For this review, use the dimensioned drawing (mm, ordinates from the lowest corner) and the shaded views. A direction names the side the tool comes from. Give positions to 0.01 mm unless a question says otherwise; leave off trailing zeros. Order: outer loops, then holes, each group sorted by start corner. A loop starts at its lowest first (then second) coordinate and runs counter-clockwise, first axis right, second up.
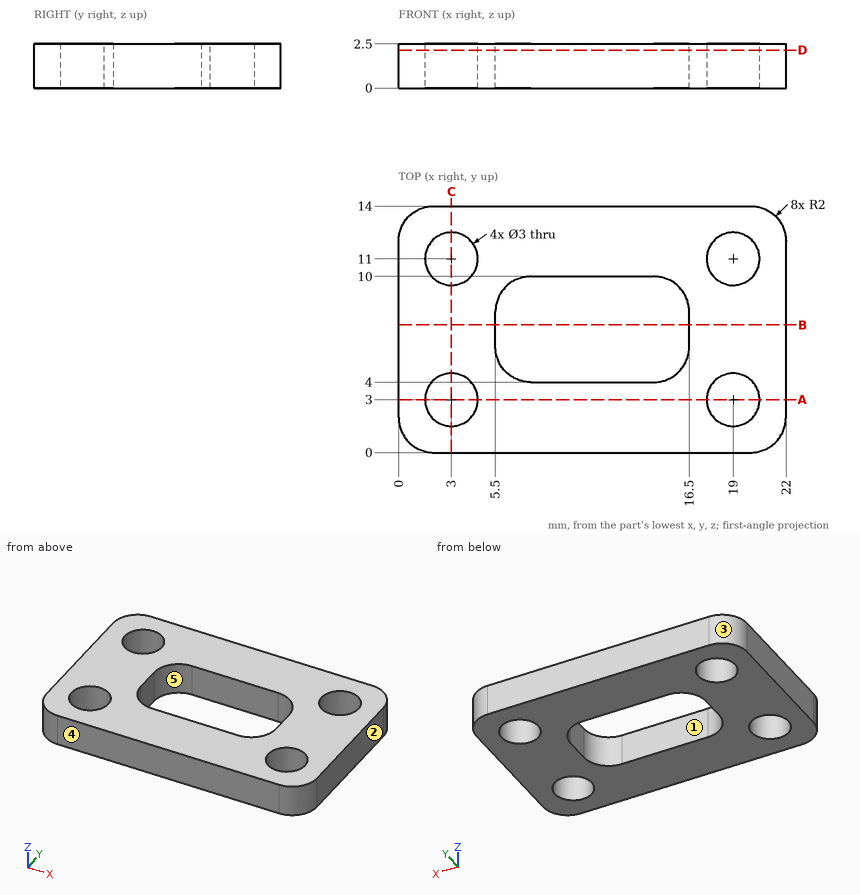
1. For pin 1 (2.5 mm diameter, centred on x = 19, y = 11, fed in from -Z); pin 2 (4 mm diameter, centred on x = 13, y = 5.5, fed in from -Z), all flat-tipped, find the tip position at first contact; note any pin that passes through.
Recorded:
pin 1: passes through
pin 2: stops at z = 0
2. Machinability: for the marked faces 1 and 2, which of the approach directions +Z, -Z, +X, -X, +Y, -Y give a long, thin tool a straight path to every point of the face, cutting with its end or side? Answer none if there is none.
Recorded:
face 1: +Z, -Z
face 2: +Z, -Z, +X, +Y, -Y
3. For line 1 along Y through (x, z) = (3, 1.55); line 2 along Y through (x, z) = (13, 0.45); line 3 along X through (y, z) = (2.5, 1.8), list the stretches that pass through material, from the lowest coordinate up.
Recorded:
line 1: y = 0 to 1.5, 4.5 to 9.5, 12.5 to 14
line 2: y = 0 to 4, 10 to 14
line 3: x = 0 to 1.59, 4.41 to 17.59, 20.41 to 22
4. Draft analysis for pull direction X (two halves, no side actions). For the marked faces 3, 4 and 5, state which applies: pulls with the +X half, pulls with the -X half, needs draft (parallel to the pull), parting line crosses it, or undercut.
Recorded:
face 3: pulls with the -X half
face 4: needs draft
face 5: undercut
5. Take a section at D-D (z = 2.15). State the section outline as (x, y) points, then the cut area to 3 significant figures.
Recorded:
outline: (0, 2) arc R2 ccw to (2, 0) - (20, 0) arc R2 ccw to (22, 2) - (22, 12) arc R2 ccw to (20, 14) - (2, 14) arc R2 ccw to (0, 12) - close; hole circle Ø3 at (3, 3); hole circle Ø3 at (3, 11); hole (5.5, 6) arc R2 ccw to (7.5, 4) - (14.5, 4) arc R2 ccw to (16.5, 6) - (16.5, 8) arc R2 ccw to (14.5, 10) - (7.5, 10) arc R2 ccw to (5.5, 8) - close; hole circle Ø3 at (19, 3); hole circle Ø3 at (19, 11)
area: 214 mm2
6. Take a section at A-A (y = 3). State the section outline as (x, z) points, then the cut area to 3 significant figures.
Recorded:
outline: (0, 0) - (1.5, 0) - (1.5, 2.5) - (0, 2.5) - close; (4.5, 0) - (17.5, 0) - (17.5, 2.5) - (4.5, 2.5) - close; (20.5, 0) - (22, 0) - (22, 2.5) - (20.5, 2.5) - close
area: 40.0 mm2
7. Take a section at B-B (y = 7.25). State the section outline as (x, z) points.
Recorded:
outline: (0, 0) - (5.5, 0) - (5.5, 2.5) - (0, 2.5) - close; (16.5, 0) - (22, 0) - (22, 2.5) - (16.5, 2.5) - close
8. Take a section at C-C (x = 3). State the section outline as (y, z) points.
Recorded:
outline: (0, 0) - (1.5, 0) - (1.5, 2.5) - (0, 2.5) - close; (4.5, 0) - (9.5, 0) - (9.5, 2.5) - (4.5, 2.5) - close; (12.5, 0) - (14, 0) - (14, 2.5) - (12.5, 2.5) - close
